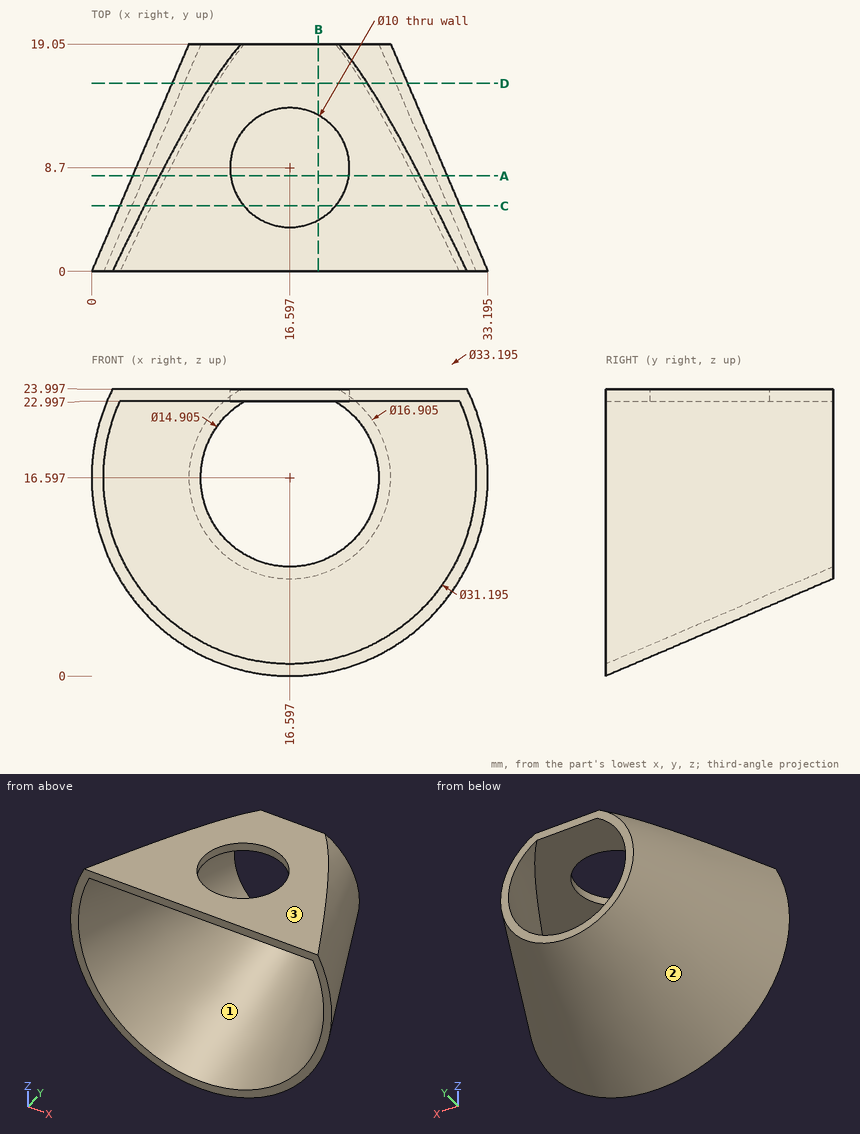
Geometry: see drawing. Coordinates: mm, zero at the bounding-box minimum. Give positions to 0.01 mm unless a question says otherwise; leave off trailing zeros. Write each loop counter-clockwise with the first axis right and the second up, starting at its lowest first coordinate (ties: lowest second). Pieces come first, ordered by that corner, then holes. Notation, with made-up numbers: M 21.25,81.5 L 38.25,81.5 A35 cw 38.25,114.5 Z; hole C -5.75,62.5 d9. An arc over 180 degrees is marked long. Answer in a Markdown table with one row per item. Add a question column.
(1) Section B-B on x = 19. State how many separate pieces and enclosed holes the cut face has.
(2) Section A-A on y = 8. Return loops of the section in (x, z) (1 decimal).
(3) First-contact query: pin 1 (1.5 mm diameter, centred on x = 24.5, z = 17.5, fed in from -Y) (1 decimal); pin 2 (2 mm diameter, centred on y = 16.5, z = 8.5, fed in from +X) (1 decimal); pin 3 (2 mm diameter, centred on y = 7.5, z = 7.5, fed in from +X). Flat tips, straight axial feed; report the tip coordinate or a pass-through.
(4) Mould query, pull axis Z, two halves, no side actions, for the marked faces 1, 2 and 3. Classes: +Z half, -Z half, draft (parallel to the pull), parting line (faces both ways), or undercut.
(5) Section D-D on y = 15.75. Return loops of the section in (x, z) (1 decimal).
(6) Ray query, line 1 (Z direction, x = 19, y = 16.5); line 2 (Z direction, x = 22, y = 9.25) (1 decimal); line 3 (X direction, y = 9.25, z = 20.5) (1 decimal). Return the intervals inside material, ascending.
(7) Section C-C on y = 5.5. Return loops of the section in (x, z) (1 decimal).
Result set:
| question | item | result |
|---|---|---|
| 1 | separate pieces | 3 |
| 1 | enclosed holes | 0 |
| 2 | outline | M 5.7,24 A13.2 ccw long 27.5,24 L 21.5,24 L 21.5,23 L 27,23 A12.2 cw long 6.2,23 L 11.6,23 L 11.6,24 Z |
| 3 | pin 1 | stops at y = 16.1 |
| 3 | pin 2 | stops at x = 23.1 |
| 3 | pin 3 | stops at x = 27.43 |
| 4 | face 1 | undercut |
| 4 | face 2 | parting line |
| 4 | face 3 | +Z half |
| 5 | outline | M 10.1,24 A9.9 ccw long 23.1,24 Z; hole M 10.5,23 A8.9 ccw long 22.7,23 Z |
| 6 | line 1 | z = 7.36 to 8.4, 23 to 24 |
| 6 | line 2 | z = 5.2 to 6.3, 23 to 24 |
| 6 | line 3 | x = 4.6 to 5.6, 27.6 to 28.6 |
| 7 | outline | M 4.4,24 A14.2 ccw long 28.8,24 L 20.4,24 L 20.4,23 L 28.2,23 A13.2 cw long 5,23 L 12.8,23 L 12.8,24 Z |
